```python
from build123d import *

# Parameters (mm, degrees)
SKETCH1_W                      = 120
SKETCH1_H                      = 111.5
BOSS_EXTRUDE1_DEPTH            = 12.7
SKETCH2_R                      = 22.5
CUT_EXTRUDE1_DEPTH             = 6.35
FILLET1_R                      = 6.35
CBORE_FOR_M5_SHCS1_D           = 5.5
CBORE_FOR_M5_SHCS1_CBORE_D     = 10
CBORE_FOR_M5_SHCS1_CBORE_DEPTH = 5
CBORE_FOR_M6_SHCS1_D           = 6.6
CBORE_FOR_M6_SHCS1_CBORE_D     = 11
CBORE_FOR_M6_SHCS1_CBORE_DEPTH = 6


with BuildPart() as part:
    # Sketch1 → Boss-Extrude1 (new body)
    with BuildSketch(Plane.XY):
        Rectangle(SKETCH1_W, SKETCH1_H)
    extrude(amount=BOSS_EXTRUDE1_DEPTH)

    # Sketch2 → Cut-Extrude1 (cut)
    with BuildSketch(Plane.XY.offset(12.7)):
        with Locations((-10.2, 17.75)):
            Circle(SKETCH2_R)
        Polygon((38.2, -8.25), (38.2, -16.75), (51.2, -16.75), (51.2, -35.75), (38.2, -35.75), (20, -35.75), (20, -55.75), (-20, -55.75), (-20, -35.75), (-28, -35.75), (-41, -35.75), (-41, -16.75), (-28, -16.75), (-28, -8.25), align=None)
    extrude(amount=-CUT_EXTRUDE1_DEPTH, mode=Mode.SUBTRACT)

    # Fillet1
    fillet1_edges = [part.edges().sort_by_distance(p)[0] for p in [
        (-28, -8.25, 9.525),
        (38.2, -8.25, 9.525),
        (51.2, -16.75, 9.525),
        (51.2, -35.75, 9.525),
        (-41, -35.75, 9.525),
        (-41, -16.75, 9.525),
    ]]
    fillet(fillet1_edges, radius=FILLET1_R)

    # CBORE for M5 SHCS1 (through all)
    with Locations(Plane(origin=(0, 0, 0), x_dir=(-1, 0, 0), z_dir=(0, 0, -1))):
        with Locations((-33.2, 30.75), (-14.8, 30.75), (-14.8, -3.25), (-43.2, -11.75), (33, -11.75)):
            CounterBoreHole(CBORE_FOR_M5_SHCS1_D / 2, CBORE_FOR_M5_SHCS1_CBORE_D / 2, CBORE_FOR_M5_SHCS1_CBORE_DEPTH)

    # CBORE for M6 SHCS1 (through all)
    with Locations(Plane.XY.offset(12.7)):
        with Locations((-50, 45.75), (50, 45.75), (50, -45.75), (-50, -45.75)):
            CounterBoreHole(CBORE_FOR_M6_SHCS1_D / 2, CBORE_FOR_M6_SHCS1_CBORE_D / 2, CBORE_FOR_M6_SHCS1_CBORE_DEPTH)


solid = part.part
```
Geometry check sheet. Reference: the model listing, model coordinates, mm. A direction names the side the tool comes from. Coordinates: 2 decimals unless noted, no trailing zeros. Order: outer loops, then holes, each group sorted by start corner. A loop starts at its lowest first (then second) coordinate and runs counter-clockwise, first axis right, second up.
Q1. Depth check by flat-ended pin: pin 1 Ø6 at (x, y) = (14.8, -3.25) entering from -Z; pin 2 Ø5 at (x, z) = (-16, 11) entering from -Y; pin 3 Ø6 at (x, y) = (50, -45.75) entering from +Z; pin 4 Ø4 at (x, y) = (32, -11.5) entering from +Z. Enter the tip coordinate at first touch or a pass-through.
Reply:
pin 1: stops at z = 5
pin 2: stops at y = -8.25
pin 3: passes through
pin 4: stops at z = 6.35
Q2. Sectioned sample at D-D on x = 33.2. Record the cut outline in (y, z).
Reply:
outline: (-55.75, 0) - (25.75, 0) - (25.75, 5) - (28, 5) - (28, 12.7) - (-8.4, 12.7) - (-8.4, 6.35) - (-35.75, 6.35) - (-35.75, 12.7) - (-55.75, 12.7) - close; (33.5, 5) - (35.75, 5) - (35.75, 0) - (55.75, 0) - (55.75, 12.7) - (33.5, 12.7) - close
Q3. Sectioned sample at B-B on z = 10. Give the number of separate pieces and of enclosed holes in the cut face, and give its area (3 significant figures).
Reply:
separate pieces: 1
enclosed holes: 10
area: 8,230 mm2
Q4. Thickness scan on probe 1 along Y at (x, z) = (43.2, 8.25); probe 2 along Y at (x, z) = (14.8, 8); probe 3 along X at (y, z) = (33, 11.5). Record the ranges inside material, lowest first.
Reply:
probe 1: y = -55.75 to -35.75, -16.75 to -14.5, -9 to 55.75
probe 2: y = -8.25 to -6, -0.5 to 28, 33.5 to 55.75
probe 3: x = -60 to -26.74, 6.34 to 13.22, 16.38 to 31.62, 34.78 to 60
Q5. Draft check along Y on faces 1 (the face through (50, 42, 6.7)), 2 (the face through (-11, 18, 6.35)). Enter one of: released by +Y, released by -Y, zero draft, split by the parting line, or undercut.
Reply:
face 1: undercut
face 2: undercut
Q6. Sectioned sample at C-C on y = -28. Record the cut outline in (x, z), and give its area (3 significant figures).
Reply:
outline: (-60, 0) - (60, 0) - (60, 12.7) - (51.2, 12.7) - (51.2, 6.35) - (-41, 6.35) - (-41, 12.7) - (-60, 12.7) - close
area: 939 mm2
Q7. Sectioned sample at A-A on x = -50. Record the cut outline in (y, z), and give its area (3 significant figures).
Reply:
outline: (-55.75, 0) - (-49.05, 0) - (-49.05, 6.7) - (-51.25, 6.7) - (-51.25, 12.7) - (-55.75, 12.7) - close; (-42.45, 0) - (42.45, 0) - (42.45, 6.7) - (40.25, 6.7) - (40.25, 12.7) - (-40.25, 12.7) - (-40.25, 6.7) - (-42.45, 6.7) - close; (49.05, 0) - (55.75, 0) - (55.75, 12.7) - (51.25, 12.7) - (51.25, 6.7) - (49.05, 6.7) - close
area: 1,200 mm2
Q8. Tool access check on faces 3 (the face through (32, -35.75, 10)), 4 (the face through (-35, -14, 5)), 5 (the face through (-35.747, -11.629, 8.904)). Record the directions out of +Z, -Z, +X, -X, +Y, -Y that give a thin tool (end or side, any length) a straight path to the whole face; none if there is none.
Reply:
face 3: +Z
face 4: -Z
face 5: +Z, -Z
